Part model, mm, in its own coordinate system. A direction names the side the tool comes from. Give positions to 0.01 mm unless a question says otherwise; leave off trailing zeros. Order: outer loops, then holes, each group sorted by start corner. A loop starts at its lowest first (then second) coordinate and runs counter-clockwise, first axis right, second up.
Autodesk Inventor part; units mm, degrees
ref_plane "Start Plane" through (0, 0, 4.5707) normal (0, 0, 1) x (1, 0, 0)
ref_plane "End Plane" through (0, 0, 110) normal (0, 0, 1) x (1, 0, 0)
ref_plane "Work Plane4" through (163.4562, 7, 154.6771) normal (0.6544, 0, -0.7562) x (-0.7562, 0, -0.6544)
ref_plane "Start Plane" through (0, 0, 4.5707) normal (0, 0, 1) x (1, 0, 0)
ref_plane "End Plane" through (0, 0, 110) normal (0, 0, 1) x (1, 0, 0)
sketch "Sketch" plane through (0, 0, 0) normal (0, 0, 1) x (1, 0, 0)
  line L0 (-10, -7) -> (-10, 7)
  line L1 (-7, 10) -> (7, 10)
  line L2 (10, 7) -> (10, -7)
  line L3 (7, -10) -> (-7, -10)
  arc A0 (-10, -7) -> (-7, -10) centre (-7, -7) ccw
  arc A1 (-7, 10) -> (-10, 7) centre (-7, 7) ccw
  arc A2 (10, 7) -> (7, 10) centre (7, 7) ccw
  arc A3 (7, -10) -> (10, -7) centre (7, -7) ccw
  arc A4 (-7, 8) -> (-8, 7) centre (-7, 7) ccw
  line L4 (-7, 8) -> (7, 8)
  arc A5 (8, 7) -> (7, 8) centre (7, 7) ccw
  line L5 (8, 7) -> (8, -7)
  arc A6 (7, -8) -> (8, -7) centre (7, -7) ccw
  line L6 (7, -8) -> (-7, -8)
  arc A7 (-8, -7) -> (-7, -8) centre (-7, -7) ccw
  line L7 (-8, -7) -> (-8, 7)
  line L8 (0, 14.8698) -> (0, -14.8698) construction
  line L9 (-14.8698, 0) -> (14.8698, 0) construction
  dimension "d7" = 3
  dimension "d10" = 20
  dimension "d11" = 20
  dimension "d12" = 2
  dimension "d15" = 10
  dimension "d16" = 10
extrude "Body" add sketch "Sketch" along normal up to surface (105.4293 mm away) from surface at 4.5707
sketch "Sketch3" plane through (0, 0, 0) normal (0, 0, 1) x (1, 0, 0)
  line L0 (0, 0) -> (10, 0)
ref_plane "Work Plane3" through (0, 0, 0) normal (0, -1, 0) x (1, 0, 0)
sketch "Sketch4" plane through (0, 0, 0) normal (0, -1, 0) x (1, 0, 0)
  line L0 (-2, 4.5707) -> (12, 4.5707)
  line L1 (-2, 110) -> (12, 110)
  dimension "d18" = 105.4293
ref_plane "Work Plane4" through (163.4562, 7, 154.6771) normal (0.6544, 0, -0.7562) x (-0.7562, 0, -0.6544)
split "Split1" plane through (163.4562, 7, 154.6771) removes the side toward (0.6544, 0, -0.7562)
sketch "Sketch5" plane through (-7, 10, 110) normal (0, 1, 0) x (1, 0, 0)
  line L0 (-3, 0) -> (-3, 105.4293)
  line L1 (4805.2907, 8171.9937) -> (4797.7312, 8176.4206)
  line L2 (-3, 29.0626) -> (17, 29.0626)
  line L3 (-3, 5.4293) -> (17, 5.4293)
  circle A0 centre (7.3777, 19.0626) radius 5
  circle A1 centre (7.3777, 19.0626) radius 5 construction
  line L4 (4797.7312, 8176.4206) -> (4800.2551, 8213.114)
  line L5 (12.3777, 19.0626) -> (12.3777, -7767.3118)
  line L6 (-3, 105.4293) -> (0, 102.8331)
  line L7 (14, 90.7177) -> (17, 88.1216)
  line L8 (0, 0) -> (14, 0)
  arc A2 (12.3777, 11.5793) -> (2.3777, 11.5793) centre (7.3777, 19.0626) ccw
  line L9 (7.3777, 19.0626) -> (7.3777, 0) construction
  line L10 (7.3777, 19.0626) -> (7.3777, 29.6702) construction
  line L11 (2.3777, 0) -> (2.3777, 19.0626)
  line L12 (17, 88.1216) -> (17, 0)
  line L13 (-3, 0) -> (17, 0)
  line L14 (0, 0) -> (-3, 0)
  point P0 (7, 110)
  point P1 (7.3777, 28.0626)
  point P2 (2.3777, 5.4293)
  point P3 (12.3777, 5.4293)
  point P4 (12.3777, 0)
  point P5 (12.3777, 11.5793)
  point P6 (2.3777, 11.5793)
  point P7 (12.3777, 19.0626)
  point P8 (17, 60.7933)
  dimension "d23" = 10
  dimension "d27" = 18
  dimension "d28" = 1
  dimension "d33" = 100
extrude "Extrusion2" cut sketch "Sketch5" against normal up to surface (18 mm away) contours L0 L3 L11 L8 L13 | L0 L2 L12 L3 L5 A2 L11 | L11 A0 L5 L3 | L3 L12 L13 L8 L5 | A2 L5 A0 L11
extrude "Extrusion3" cut sketch "Sketch5" against normal through all contours L0 L3 L11 L8 L13 | L11 A0 L5 L3 | L3 L5 L8 L11 | L3 L12 L13 L8 L5 | A0
equation "\"d7\" = G_IR"
equation "\"d10\" = G_H"
equation "\"d11\" = G_W"
equation "\"d12\" = G_T"
equation "\"d15\" = 0.5 * d10"
equation "\"d16\" = 0.5 * d11"
equation "\"d3\" = G_L"
equation "\"G_W\" = 20"
equation "\"G_H\" = 20"
equation "\"G_T\" = 2"
equation "\"G_IR\" = 3"
equation "\"G_L\" = d18"
equation "\"G_OFFSET_START\" = -4.57072"
equation "\"G_OFFSET_END\" = 0"
equation "\"d13\" = -G_OFFSET_START"
properties part number "ISO 12633-2 - 20x20x2 - 105,43" material "Steel, Mild"
Item 1: Band-saw the part on D-D on z = 18. List the corners of the cut face in (x, y).
Item 2: Band-saw the part on A-A on y = -6. List the corners of the cut face in (x, z).
Item 3: Band-saw the part on B-B on x = 1.25. List the corners of the cut face in (y, z), plus the area to 3 significant figures.
Item 4: Which spindle directions (+Z, -Z, +X, -X, +Y, -Y) get a long thin tool onto all of the face, cutting with end or side? Do faces 1 (the face through (-9.1, -9.14, 53.87)), 2 (the face through (5.378, -9, 98)), 3 (the face through (0, 8.4, 80.937)), 4 (the face through (-8, 0, 43)). Say none if no direction does.
Item 5: Band-saw the part on C-C on z = 64. List the corners of the cut face in (x, y).
Item 6: Drop a flat-ended pin along its axis: P1, Ø0.6, axis at y = -9, z = 99, coming from the +X side. Give the stop position or say it passes through.
Item 7: Pull direction X, two halves, no side cores. Call faces 5 (the face through (0.49, -8.99, 85.94)), 6 (the face through (0, 10, 44)), 7 (the face through (9.14, -9.1, 61.33)), 8 (the face through (8, 0, 50)): released by +X, released by -X, zero draft, split by the parting line, or undercut.
Item 8: Drill centre lines: probe 1 along Y at (x, z) = (2, 77); probe 2 along Y at (x, z) = (-7, 88.5). Where is each one in solid material? Low to high.
Working result:
1. outline: (-10, -7) arc R3 ccw to (-7, -10) - (5.52, -10) - (5.52, -8) - (-7, -8) arc R1 cw to (-8, -7) - (-8, 7) arc R1 cw to (-7, 8) - (5.52, 8) - (5.52, 10) - (-7, 10) arc R3 ccw to (-10, 7) - close
2. outline: (-10, 4.57) - (-8, 6.3) - (-8, 80.94) - (-10, 80.94) - close; (8, 20.15) - (10, 21.88) - (10, 80.94) - (8, 80.94) - close
3. outline: (-10, 14.31) - (-8, 14.31) - (-8, 86.01) - (-10, 86.01) - close; (8, 14.31) - (10, 14.31) - (10, 80.94) - (8, 80.94) - close
3. area: 277 mm2
4. face 1: +Z, -Z, -X, -Y
4. face 2: +Z, +Y, -Y
4. face 3: +Z, +X, -X, +Y
4. face 4: +Z, -Z
5. outline: (-10, -7) arc R3 ccw to (-7, -10) - (7, -10) arc R3 ccw to (10, -7) - (10, 7) arc R3 ccw to (7, 10) - (-7, 10) arc R3 ccw to (-10, 7) - close; hole (-8, -7) arc R1 ccw to (-7, -8) - (7, -8) arc R1 ccw to (8, -7) - (8, 7) arc R1 ccw to (7, 8) - (-7, 8) arc R1 ccw to (-8, 7) - close
6. P1: stops at x = 9.47
7. face 5: undercut
7. face 6: zero draft
7. face 7: released by +X
7. face 8: undercut
8. probe 1: y = -10 to -8, 8 to 10
8. probe 2: y = -10 to -8
